Part model, mm, in its own coordinate system. A direction names the side the tool comes from. Round coordinates to 2 decimals unless told otherwise and drop trailing zeros. Write each loop counter-clockwise with the first axis right and the second up, starting at its lowest first coordinate (ties: lowest second). Pieces come first, ordered by that corner, then holes. Notation, with made-up numbers: M 59.5,-31.5 L 108.5,-31.5 A22 ccw 108.5,2.5 Z; hole C 86,22 d6. An arc over 180 degrees is marked long. Use one line per item in the form item = value. Start each with the question number.
Item 1: Which spindle directions (+Z, -Z, +X, -X, +Y, -Y) get a long thin tool onto all of the face, cutting with end or side? Do faces 4 (the face through (18.72, -1.99, 10.83)), 5 (the face through (-38, -5, -1)), 6 (the face through (38, -5, -1)), 7 (the face through (-30.01, -0.49, -29.85)), 8 (the face through (-4.23, -5.46, 22.85)). Say none if no direction does.
Item 2: Cut at C-C, the plane x = -33. Give the cut face in (y, z).
Item 3: Cut at B-B, the plane x = -7. Give the cut face in (y, z), then the cut area to 3 significant figures.
Item 4: Flat gauge pins, fed straight in: pin 1 Ø2.5 at (y, z) = (-6, -12.5) entering from -X; pin 2 Ø2.5 at (x, y) = (-19, -4.5) entering from +Z; pin 3 Ø2 at (x, y) = (-29, -11) entering from +Z. Where does each tip first touch, or does it go through?
Item 5: Mould opens along Z. For faces 1 (the face through (31.62, -6.41, -35.15)), 2 (the face through (-1, -5, -38)), 3 (the face through (-39, 0, 3)) say: +Z half, -Z half, draft (parallel to the pull), parting line (faces both ways), or undercut.
Item 6: Probe L1, parallel to X at y = -7, z = -14.5; L2, parallel to Z at x = -7, y = -4.2; L3, parallel to X at y = -7, z = -18.5. List the from-to ranges inside material, lowest first.
Item 7: Cut at D-D, the plane x = 3. Give the cut face in (y, z), then the cut area to 3 significant figures.
Item 8: Cut at A-A, the plane z = 24. Give the cut face in (x, y).
from build123d import *

# Parameters (mm, degrees)
SKETCH2_W           = 80
SKETCH2_H           = 80
BOSS_EXTRUDE1_DEPTH = 3
CUT_EXTRUDE1_DEPTH  = 1
SKETCH5_W           = 76
SKETCH5_H           = 76
BOSS_EXTRUDE2_DEPTH = 5
SKETCH6_W           = 74
SKETCH6_H           = 74
CUT_EXTRUDE2_DEPTH  = 5
SKETCH7_R           = 4.5
BOSS_EXTRUDE3_DEPTH = 10
SKETCH4_R           = 2.5
CUT_EXTRUDE8_DEPTH  = 13
SKETCH9_R           = 3
SKETCH9_R_2         = 2
BOSS_EXTRUDE4_DEPTH = 5
BOSS_EXTRUDE5_DEPTH = 5
CUT_EXTRUDE9_DEPTH  = 10


with BuildPart() as part:
    # Sketch2 → Boss-Extrude1 (new body)
    with BuildSketch(Plane(origin=(0, 0, 0), x_dir=(1, 0, 0), z_dir=(0, 1, 0))):
        Rectangle(SKETCH2_W, SKETCH2_H)
    extrude(amount=-BOSS_EXTRUDE1_DEPTH)

    # Sketch3 → Cut-Extrude1 (cut)
    with BuildSketch(Plane(origin=(0, 0, 0), x_dir=(1, 0, 0), z_dir=(0, 1, 0))):
        with BuildLine():
            Line((-27, 37), (27, 37))
            ThreePointArc((27, 37), (29.928932188, 29.928932188), (37, 27))
            Line((37, 27), (37, -27))
            ThreePointArc((37, -27), (29.928932188, -29.928932188), (27, -37))
            Line((27, -37), (-27, -37))
            ThreePointArc((-27, -37), (-29.928932188, -29.928932188), (-37, -27))
            Line((-37, -27), (-37, 27))
            ThreePointArc((-37, 27), (-29.928932188, 29.928932188), (-27, 37))
        make_face()
    extrude(amount=-CUT_EXTRUDE1_DEPTH, mode=Mode.SUBTRACT)

    # Sketch5 → Boss-Extrude2 (add)
    with BuildSketch(Plane.XZ.offset(3)):
        Rectangle(SKETCH5_W, SKETCH5_H)
    extrude(amount=BOSS_EXTRUDE2_DEPTH)

    # Sketch6 → Cut-Extrude2 (cut)
    with BuildSketch(Plane.XZ.offset(8)):
        Rectangle(SKETCH6_W, SKETCH6_H)
    extrude(amount=-CUT_EXTRUDE2_DEPTH, mode=Mode.SUBTRACT)

    # Sketch7 → Boss-Extrude3 (add)
    with BuildSketch(Plane.XZ.offset(3)):
        with Locations((-33.464466094, 33.46446609)):
            Circle(SKETCH7_R)
        with Locations((33.46446609, 33.46446609)):
            Circle(SKETCH7_R)
        with Locations((-33.464466094, -33.464466094)):
            Circle(SKETCH7_R)
        with Locations((33.46446609, -33.464466094)):
            Circle(SKETCH7_R)
    extrude(amount=BOSS_EXTRUDE3_DEPTH)

    # Sketch4 → Cut-Extrude8 (cut)
    with BuildSketch(Plane(origin=(0, 0, 0), x_dir=(1, 0, 0), z_dir=(0, 1, 0))):
        with Locations((33.46446609, 33.464466094)):
            Circle(SKETCH4_R)
        with Locations((-33.464466094, 33.464466094)):
            Circle(SKETCH4_R)
        with Locations((-33.464466094, -33.46446609)):
            Circle(SKETCH4_R)
        with Locations((33.46446609, -33.46446609)):
            Circle(SKETCH4_R)
    extrude(amount=-CUT_EXTRUDE8_DEPTH, mode=Mode.SUBTRACT)

    # Sketch9 → Boss-Extrude4 (add)
    with BuildSketch(Plane.XZ.offset(3)):
        with Locations((-7, 24)):
            Circle(SKETCH9_R)
        with Locations((-7, 24)):
            Circle(SKETCH9_R_2, mode=Mode.SUBTRACT)
    extrude(amount=BOSS_EXTRUDE4_DEPTH)

    # Sketch10 → Boss-Extrude5 (add)
    with BuildSketch(Plane.XZ.offset(3)):
        with BuildLine():
            Line((-8.5, -10), (-8.5, -17))
            ThreePointArc((-8.5, -17), (-9, -17.5), (-9.5, -17))
            Line((-9.5, -17), (-9.5, -10))
            ThreePointArc((-9.5, -10), (-9, -9.5), (-8.5, -10))
        make_face()
        with BuildLine():
            Line((13, -10), (13, -17))
            ThreePointArc((13, -17), (12.5, -17.5), (12, -17))
            Line((12, -17), (12, -10))
            ThreePointArc((12, -10), (12.5, -9.5), (13, -10))
        make_face()
    extrude(amount=BOSS_EXTRUDE5_DEPTH)

    # Sketch11 → Cut-Extrude9 (cut)
    with BuildSketch(Plane(origin=(0, -1, 0), x_dir=(1, 0, 0), z_dir=(0, 1, 0))):
        Polygon((17.300412364, -3.292028925), (11.526909672, -3.292028925), (8.640158326, -8.292028925), (11.526909672, -13.292028925), (17.300412364, -13.292028925), (20.18716371, -8.292028925), align=None)
    extrude(amount=-CUT_EXTRUDE9_DEPTH, mode=Mode.SUBTRACT)


solid = part.part
Model answer:
q1.face_4 = +Y, -Y
q1.face_5 = +Z, -Z, -X, -Y
q1.face_6 = +Z, -Z, +X, -Y
q1.face_7 = +Y
q1.face_8 = -Y
q2.outline = M -13,-37.94 L -8,-37.94 L -8,-38 L -3,-38 L -3,-40 L 0,-40 L 0,-35.92 L -13,-35.92 Z; M -13,-31.01 L 0,-31.01 L 0,-27.83 L -1,-27.83 L -1,27.83 L 0,27.83 L 0,31.01 L -13,31.01 L -13,28.99 L -3,28.99 L -3,-28.99 L -13,-28.99 Z; M -13,35.92 L 0,35.92 L 0,40 L -3,40 L -3,38 L -8,38 L -8,37.94 L -13,37.94 Z
q3.outline = M -8,-38 L -3,-38 L -3,-40 L 0,-40 L 0,-37 L -1,-37 L -1,37 L 0,37 L 0,40 L -3,40 L -3,38 L -8,38 L -8,37 L -3,37 L -3,27 L -8,27 L -8,26 L -3,26 L -3,22 L -8,22 L -8,21 L -3,21 L -3,-37 L -8,-37 Z
q3.area = 186 mm²
q4.pin_1 = -38
q4.pin_2 = 38
q4.pin_3 = 36.34
q5.face_1 = undercut
q5.face_2 = -Z half
q5.face_3 = draft
q6.L1 = -38 to -37, -9.5 to -8.5, 12 to 13, 37 to 38
q6.L2 = -38 to -37, 21 to 22, 26 to 27, 37 to 38
q6.L3 = -38 to -37, 37 to 38
q7.outline = M -8,-38 L -3,-38 L -3,-40 L 0,-40 L 0,-37 L -1,-37 L -1,37 L 0,37 L 0,40 L -3,40 L -3,38 L -8,38 L -8,37 L -3,37 L -3,-37 L -8,-37 Z
q7.area = 176 mm²
q8.outline = M -40,-3 L -38,-3 L -38,-8 L -37,-8 L -37,-3 L -10,-3 L -10,-8 L -9,-8 L -9,-3 L -5,-3 L -5,-8 L -4,-8 L -4,-3 L 37,-3 L 37,-8 L 38,-8 L 38,-3 L 40,-3 L 40,0 L 37,0 L 37,-1 L -37,-1 L -37,0 L -40,0 Z
